Read the model definition and answer for the solid it produces. Units are mm, in the model's axes. Face numbers are marked on the shaded views. A direction names the side the tool comes from. Round coordinates to 2 decimals unless told otherwise and drop trailing zeros. Order: outer loops, then holes, each group sorted by start corner. A loop starts at its lowest first (then second) coordinate and runs counter-clockwise, first axis right, second up. Notation, with made-up numbers: (46, 45.25) - (85, 45.25) arc R38 ccw to (85, 84.25) - close; hole circle Ø2 at (42.25, 88). An arc over 180 degrees is marked (long way). Answer as a JSON object with one key per item and string values. Group by question number.
Q1. A cutting plane is placed at C-C on y = 9.25. Determine the outline of the cut face in (x, z).
Q2. Given pin 1 Ø8 at (y, z) = (5, -5.5) entering from -X; pin 2 Ø1 at (x, z) = (-7, 12) entering from -Y; pin 3 Ø13.5 at (x, z) = (-4, 1) entering from +Y; pin 4 Ø3 at (x, y) = (6, 5) entering from -Z, each flat-ended and moving along its own axis, determine where each tip first touches the part or whether it passes through.
Q3. A cutting plane is placed at D-D on x = 0. Determine the outline of the cut face in (y, z).
Q4. Consider line 1 (Y direction, x = 1, z = -5); line 2 (Z direction, x = -12.75, y = 5.5); line 3 (Z direction, x = 0.25, y = 1.5). Determine where each line is inside the solid, lowest interval first.
Q5. A cutting plane is placed at A-A on x = -6. Determine the outline of the cut face in (y, z).
Q6. A cutting plane is placed at B-B on z = 2. Determine the outline of the cut face in (x, y), and give its area (3 significant figures).
Q7. A tool of negligible diameter and unlimited length cuts with its end or side. For the marked faces 1 and 2, from which of +Z, -Z, +X, -X, +Y, -Y can it reach the whole face along a straight path? Write none if from no direction.
```python
from build123d import *

# Parameters (mm, degrees)
BOSS_EXTRUDE1_DEPTH = 3
BOSS_EXTRUDE2_DEPTH = 15.5


with BuildPart() as part:
    # Sketch1 → Boss-Extrude1 (new body)
    with BuildSketch(Plane(origin=(0, 0, 0), x_dir=(1, 0, 0), z_dir=(0, 1, 0))):
        with BuildLine():
            Line((-10, 0), (-14, -25))
            Line((-14, -25), (14, -25))
            Line((14, -25), (10, 0))
            ThreePointArc((10, 0), (0, 10), (-10, 0))
        make_face()
    extrude(amount=BOSS_EXTRUDE1_DEPTH)

    # Sketch5 → Boss-Extrude2 (add)
    with BuildSketch(Plane(origin=(0, 3, 0), x_dir=(1, 0, 0), z_dir=(0, 1, 0))):
        Polygon((-13.52, -22), (13.52, -22), (14, -25), (-14, -25), align=None)
    extrude(amount=BOSS_EXTRUDE2_DEPTH)


solid = part.part
```
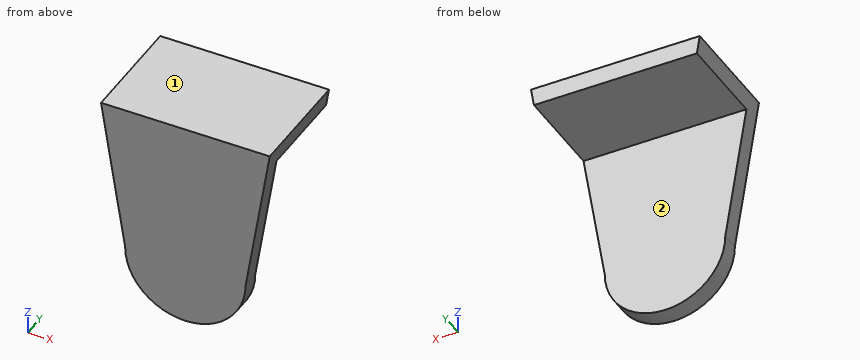
Result set:
{
 "1": {"outline": "(-14, 25) - (-13.52, 22) - (13.52, 22) - (14, 25) - close"},
 "2": {"pin 1": "stops at x = -9.79", "pin 2": "stops at y = 0", "pin 3": "stops at y = 3", "pin 4": "stops at z = 22"},
 "3": {"outline": "(0, -10) - (3, -10) - (3, 22) - (18.5, 22) - (18.5, 25) - (0, 25) - close"},
 "4": {"line 1": "y = 0 to 3", "line 2": "z = 22 to 25", "line 3": "z = -10 to 25"},
 "5": {"outline": "(0, -8) - (3, -8) - (3, 22) - (18.5, 22) - (18.5, 25) - (0, 25) - close"},
 "6": {"outline": "(-10.32, 0) - (10.32, 0) - (10.32, 3) - (-10.32, 3) - close", "area": "61.9 mm²"},
 "7": {"face 1": "+Z, +X, -X, +Y, -Y", "face 2": "-Z, +X, -X, +Y"}
}
